from build123d import *

# Parameters (mm, degrees)
SKETCH1_W           = 54
SKETCH1_H           = 30
BOSS_EXTRUDE1_DEPTH = 5
SKETCH2_W           = 54
SKETCH2_H           = 5
BOSS_EXTRUDE2_DEPTH = 36
SKETCH3_W           = 7
SKETCH3_H           = 20
BOSS_EXTRUDE3_DEPTH = 10
SKETCH6_W           = 7
SKETCH6_H           = 30
CUT_EXTRUDE2_DEPTH  = 36
SKETCH7_R           = 1.5
CUT_EXTRUDE3_DEPTH  = 5
BOSS_EXTRUDE4_DEPTH = 9
FILLET1_R           = 10


with BuildPart() as part:
    # Sketch1 → Boss-Extrude1 (new body)
    with BuildSketch(Plane(origin=(0, 0, 0), x_dir=(1, 0, 0), z_dir=(0, 1, 0))):
        with Locations((27, 15)):
            Rectangle(SKETCH1_W, SKETCH1_H)
    extrude(amount=BOSS_EXTRUDE1_DEPTH)

    # Sketch2 → Boss-Extrude2 (add)
    with BuildSketch(Plane(origin=(0, 5, 0), x_dir=(1, 0, 0), z_dir=(0, 1, 0))):
        with Locations((27, 27.5)):
            Rectangle(SKETCH2_W, SKETCH2_H)
        with Locations((27, 2.5)):
            Rectangle(SKETCH2_W, SKETCH2_H)
    extrude(amount=BOSS_EXTRUDE2_DEPTH)

    # Sketch3 → Boss-Extrude3 (add)
    with BuildSketch(Plane(origin=(0, 41, 0), x_dir=(1, 0, 0), z_dir=(0, 1, 0))):
        with Locations((50.5, 15)):
            Rectangle(SKETCH3_W, SKETCH3_H)
    extrude(amount=-BOSS_EXTRUDE3_DEPTH)

    # Sketch6 → Cut-Extrude2 (cut)
    with BuildSketch(Plane.XZ):
        with Locations((50.5, -15)):
            Rectangle(SKETCH6_W, SKETCH6_H)
    extrude(amount=-CUT_EXTRUDE2_DEPTH, mode=Mode.SUBTRACT)

    # Sketch7 → Cut-Extrude3 (cut)
    with BuildSketch(Plane.ZY):
        with Locations((-27.5, 5)):
            Circle(SKETCH7_R)
        with Locations((-2.5, 5)):
            Circle(SKETCH7_R)
    extrude(amount=-CUT_EXTRUDE3_DEPTH, mode=Mode.SUBTRACT)

    # Sketch8 → Boss-Extrude4 (add)
    with BuildSketch(Plane(origin=(0, 41, 0), x_dir=(1, 0, 0), z_dir=(0, 1, 0))):
        with BuildLine():
            Line((22.738593384, 25), (29.6, 25))
            ThreePointArc((29.6, 25), (49.6, 15), (29.6, 5))
            Line((29.6, 5), (22.738593384, 5))
            ThreePointArc((22.738593384, 5), (54.6, 15), (22.738593384, 25))
        make_face()
    extrude(amount=BOSS_EXTRUDE4_DEPTH)

    # Fillet1
    # the kernel refuses this fillet: 10 mm, written as the material it adds along each edge
    with BuildSketch(Plane(origin=(3.086121811, 41, 0), x_dir=(0, -1, 0), z_dir=(1, 0, 0))) as fillet1_piece_1_section:
        with BuildLine():
            CenterArc((FILLET1_R, -FILLET1_R), FILLET1_R, 90, 90)
            Line((0, -FILLET1_R), (0, 0))
            Line((0, 0), (FILLET1_R, 0))
        make_face()
    fillet1_piece_1 = extrude(amount=68.027756377, mode=Mode.PRIVATE)
    fillet1_piece_1 = fillet1_piece_1 & Plane(origin=(37.1, 34.728997309, -15), x_dir=(-0.82065180664829, 0, 0.5714285714285713), z_dir=(0, -1, 0)) * Cylinder(17.5, 177, mode=Mode.PRIVATE)
    add(fillet1_piece_1)
    with BuildSketch(Plane(origin=(3.086121811, 41, -30), x_dir=(0, -1, 0), z_dir=(1, 0, 0))) as fillet1_piece_2_section:
        with BuildLine():
            CenterArc((FILLET1_R, FILLET1_R), FILLET1_R, 180, 90)
            Line((0, FILLET1_R), (0, 0))
            Line((0, 0), (FILLET1_R, 0))
        make_face()
    fillet1_piece_2 = extrude(amount=68.027756377, mode=Mode.PRIVATE)
    fillet1_piece_2 = fillet1_piece_2 & Plane(origin=(37.1, 34.728997309, -15), x_dir=(-0.82065180664829, 0, 0.5714285714285713), z_dir=(0, -1, 0)) * Cylinder(17.5, 177, mode=Mode.PRIVATE)
    add(fillet1_piece_2)


solid = part.part
Verification items for the finished model (mm, model axes). A direction names the side the tool comes from. Coordinates: 2 decimals unless noted, no trailing zeros. Loops run counter-clockwise (first coordinate to the right, second up) from the corner with the lowest first, then second, coordinate; pieces in that order, holes last. Notation, with made-up numbers: (19, -17) -> (42, -17) arc R16 cw to (42, 14) -> close; hole circle Ø7 at (53, 70.5). An arc over 180 degrees is marked (long way). Answer as a JSON object with one key per item and string values. Group by question number.
Item 1: Sectioned sample at A-A on y = 8. Record the boundary of the cut face in (x, z), plus the area to 3 significant figures.
Item 2: Sectioned sample at B-B on z = -13. Record the boundary of the cut face in (x, y).
Item 3: Sectioned sample at C-C on x = 37.1. Record the boundary of the cut face in (y, z).
Item 4: Tool access check on faces 4 (the flat face through (48, 41, -15)), 5 (the flat face through (14, 41, -28)), 6 (the flat face through (37, 41, -26)). Record the directions out of +Z, -Z, +X, -X, +Y, -Y that give a thin tool (end or side, any length) a straight path to the whole face; none if there is none.
Item 5: Scan lines: probe 1 along Z at (x, y) = (22.5, 20.5); probe 2 along Z at (x, y) = (37.1, 47.5); probe 3 along Y at (x, z) = (2.15, -2.5). Record each from-to range of solid material in increasing order.
Item 6: Mould release check, pull along Z, two halves, no side actions. Record for faces 1 (the cylindrical face through (49.594, 45.437, -15.387)), 2 (the flat face through (21, 20, -30)), 3 (the flat face through (21, 20, 0)): +Z half, -Z half, draft (parallel to the pull), parting line (faces both ways), or undercut.
Item 7: Sectioned sample at D-D on z = -6.5. Record the boundary of the cut face in (x, y).
Item 8: Depth check by flat-ended pin: pin 1 (2.5 mm diameter, centred on y = 5, z = -2.5, fed in from -X); pin 2 (6 mm diameter, centred on x = 42.5, y = 36.5, fed in from -Z) (3 decimals); pin 3 (0.5 mm diameter, centred on x = 54, z = -15, fed in from -Y). Enter the tip coordinate at first touch or a pass-through.
Evaluation:
{
 "1": {"outline": "(0, -30) -> (47, -30) -> (47, -25) -> (0, -25) -> close; (0, -5) -> (47, -5) -> (47, 0) -> (0, 0) -> close", "area": "470 mm²"},
 "2": {"outline": "(0, 0) -> (47, 0) -> (47, 5) -> (0, 5) -> close; (47, 36) -> (54, 36) -> (54, 41) -> (54.49, 41) -> (54.49, 50) -> (49.44, 50) -> (49.44, 41) -> (47, 41) -> close"},
 "3": {"outline": "(0, -30) -> (31, -30) arc R10 cw to (37.61, -32.5) -> (50, -32.5) -> (50, -27.5) -> (41, -27.5) -> (41, -25) -> (5, -25) -> (5, -5) -> (41, -5) -> (41, -2.5) -> (50, -2.5) -> (50, 2.5) -> (37.61, 2.5) arc R10 cw to (31, 0) -> (0, 0) -> close"},
 "4": {"face 4": "-X, +Y", "face 5": "-Z, -X, +Y", "face 6": "+Y"},
 "5": {"probe 1": "z = -30 to -25, -5 to 0", "probe 2": "z = -32.5 to -27.5, -2.5 to 2.5", "probe 3": "y = 0 to 3.5, 6.5 to 41"},
 "6": {"face 1": "undercut", "face 2": "-Z half", "face 3": "+Z half"},
 "7": {"outline": "(0, 0) -> (47, 0) -> (47, 5) -> (0, 5) -> close; (46.27, 41) -> (47, 41) -> (47, 36) -> (54, 36) -> (54, 41) -> (52.4, 41) -> (52.4, 50) -> (46.27, 50) -> close"},
 "8": {"pin 1": "stops at x = 5", "pin 2": "stops at z = -32.315", "pin 3": "stops at y = 36"}
}
